```python
from build123d import *

# Parameters (mm, degrees)
F1_DEPTH = 20
F3_DEPTH = 15
F4_SIZE  = 3
F5_W     = 3
F5_H     = 10
F6_DEPTH = 10
F7_W     = 3
F7_H     = 6
F8_DEPTH = 25
F9_R     = 2
F10_SIZE = 2


with BuildPart() as f1:
    # F0 (on Top) → F1 (new body)
    with BuildSketch(Plane.XY):
        Polygon((5, 10), (-5, 10), (-5, -10), (5, -10), (5, -3), (6.5, -3), (6.5, 3), (5, 3), align=None)
    extrude(amount=F1_DEPTH)

    # F2 (on face) → F3 (cut)
    with BuildSketch(Plane.YZ.offset(6.5)):
        with BuildLine():
            ThreePointArc((3, 8.1972243623), (3.3726843908, 9.0645856533), (3.5, 10))
            ThreePointArc((3.5, 10), (3.3726843908, 10.9354143467), (3, 11.8027756377))
            Line((3, 11.8027756377), (3, 8.1972243623))
        make_face()
        with BuildLine():
            Line((3, 8.1972243623), (3, 11.8027756377))
            ThreePointArc((3, 11.8027756377), (0, 13.5), (-3, 11.8027756377))
            Line((-3, 11.8027756377), (-3, 8.1972243623))
            ThreePointArc((-3, 8.1972243623), (0, 6.5), (3, 8.1972243623))
        make_face()
        with BuildLine():
            Line((-3, 8.1972243623), (-3, 11.8027756377))
            ThreePointArc((-3, 11.8027756377), (-3.5, 10), (-3, 8.1972243623))
        make_face()
    extrude(amount=-F3_DEPTH, mode=Mode.SUBTRACT)

    # F4
    f4_edges = [f1.edges().sort_by_distance(p)[0] for p in [
        (-5, 3, 8.197224),
    ]]
    chamfer(f4_edges, length=F4_SIZE)

    # F5 (on face) → F6 (join)
    with BuildSketch(Plane(origin=(-5, 0, 0), x_dir=(0, -1, 0), z_dir=(-1, 0, 0))):
        with Locations((8.5, 5)):
            Rectangle(F5_W, F5_H)
        with Locations((-8.5, 5)):
            Rectangle(F5_W, F5_H)
    extrude(amount=F6_DEPTH)

    # F7 (on face) → F8 (cut)
    with BuildSketch(Plane.XZ.offset(10)):
        with Locations((-11.3098823801, 5)):
            Rectangle(F7_W, F7_H)
    extrude(amount=-F8_DEPTH, mode=Mode.SUBTRACT)

    # F9
    f9_edges = [f1.edges().sort_by_distance(p)[0] for p in [
        (-5, -10, 15),
        (-5, 10, 15),
    ]]
    fillet(f9_edges, radius=F9_R)

    # F10
    f10_edges = [f1.edges().sort_by_distance(p)[0] for p in [
        (-15, -8.5, 10),
        (-15, 8.5, 10),
        (-15, 8.5, 0),
        (-15, -8.5, 0),
        (-5, 0, 0),
        (-5, 0, 20),
    ]]
    chamfer(f10_edges, length=F10_SIZE)


solid = f1.part
```
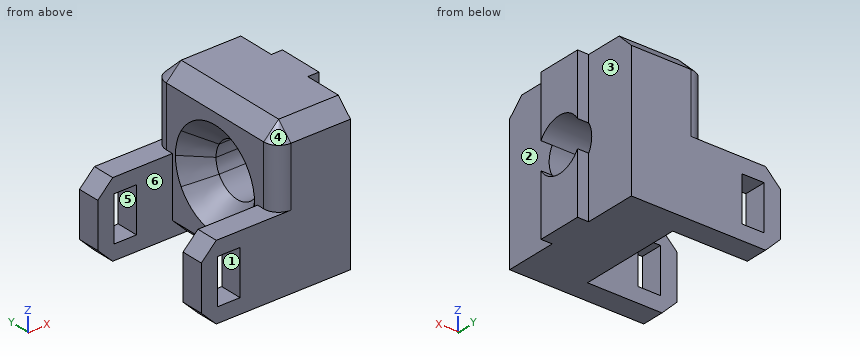
Input: part model. Units: mm. Frame: model coordinates. Face numbers are marked on the shaded views. A direction names the side the tool comes from. Round coordinates to 2 decimals unless told otherwise and drop trailing zeros. Loops run counter-clockwise (first coordinate to the right, second up) from the corner with the lowest first, then second, coordinate; pieces in that order, holes last. Notation, with made-up numbers: (63, 1.25) -> (109, 1.25) arc R18 cw to (109, 20.25) -> close; hole circle Ø4 at (-39.75, -23). An arc over 180 degrees is marked (long way). Use one line per item in the form item = value. Start each with the question number.
Item 1: Mould query, pull axis Y, two halves, no side actions, for the marked faces 4, 5 and 6. Classes: pulls with the +Y half, pulls with the -Y half, needs draft (parallel to the pull), parting line crosses it, or undercut.
Item 2: Section query D-D on x = -12.25. Return the cut outline in (y, z).
Item 3: Section query B-B on x = -7.25. Return the cut outline in (y, z), then the cut area to 3 significant figures.
Item 4: Section query A-A on z = 2.5. Return the cut outline in (x, y), then the cut area to 3 significant figures.
Item 5: Set-up query: the marked faces 1, 2 and 3. Return all of +Z, -Z, +X, -X, +Y, -Y with unobstructed straight access to the full face (end or side cutting, diameter ignored); none if empty.
Item 6: Material intervals for L1, parallel to Y at x = -7.25, z = 5; L2, parallel to X at y = 9.25, z = 4.75; L3, parallel to Y at x = 2.5, z = 13, sorted ascending. Write a range as from..to.
Item 7: Section query C-C on y = 7.5. Return the cut outline in (x, z), then the cut area to 3 significant figures.
Item 8: Contact query for flat-ended pins moving along their axis: pin 1 Ø8 at (y, z) = (-2, 3) entering from -X; pin 2 Ø5 at (y, z) = (1.5, 13) entering from -X; pin 3 Ø3.5 at (y, z) = (7.5, 5.5) entering from +X. Output: stop coordinate, or through.
Ans:
q1.face_4 = pulls with the -Y half
q1.face_5 = needs draft
q1.face_6 = undercut
q2.outline = (-10, 0) -> (-7, 0) -> (-7, 2) -> (-10, 2) -> close; (-10, 8) -> (-7, 8) -> (-7, 10) -> (-10, 10) -> close; (7, 0) -> (10, 0) -> (10, 2) -> (7, 2) -> close; (7, 8) -> (10, 8) -> (10, 10) -> (7, 10) -> close
q3.outline = (-10, 0) -> (-7, 0) -> (-7, 10) -> (-10, 10) -> close; (7, 0) -> (10, 0) -> (10, 10) -> (7, 10) -> close
q3.area = 60.0 mm^2
q4.outline = (-15, -10) -> (-12.81, -10) -> (-12.81, -7) -> (-15, -7) -> close; (-15, 7) -> (-12.81, 7) -> (-12.81, 10) -> (-15, 10) -> close; (-9.81, -10) -> (5, -10) -> (5, -3) -> (6.5, -3) -> (6.5, 3) -> (5, 3) -> (5, 10) -> (-9.81, 10) -> (-9.81, 7) -> (-5, 7) -> (-5, -7) -> (-9.81, -7) -> close
q4.area = 251 mm^2
q5.face_1 = +Y, -Y
q5.face_2 = +Z, -Z, +X, -Y
q5.face_3 = +Z, -Z, +X, +Y
q6.L1 = -10..-7, 7..10
q6.L2 = -15..-12.81, -9.81..5
q6.L3 = -10..-1.8, 1.8..10
q7.outline = (-15, 2) -> (-13, 0) -> (5, 0) -> (5, 20) -> (-3, 20) -> (-5, 18) -> (-5, 10) -> (-13, 10) -> (-15, 8) -> close; hole (-12.81, 2) -> (-9.81, 2) -> (-9.81, 8) -> (-12.81, 8) -> close
q7.area = 276 mm^2
q8.pin_1 = -5
q8.pin_2 = -4.35
q8.pin_3 = 5
